from build123d import *

# Parameters (mm, degrees)
SKETCH1_W           = 330.2
SKETCH1_H           = 25.4
BOSS_EXTRUDE4_DEPTH = 50.8
SKETCH5_W           = 19.05
SKETCH5_H           = 44.45
CUT_EXTRUDE1_DEPTH  = 330.2
SKETCH7_W           = 25.4
SKETCH7_H           = 44.45
CUT_EXTRUDE4_DEPTH  = 31.496


with BuildPart() as part:
    # Sketch1 → Boss-Extrude4 (new body)
    with BuildSketch(Plane(origin=(0, 0, 0), x_dir=(1, 0, 0), z_dir=(0, 1, 0))):
        with Locations((-165.1, -12.7)):
            Rectangle(SKETCH1_W, SKETCH1_H)
    extrude(amount=BOSS_EXTRUDE4_DEPTH)

    # Sketch5 → Cut-Extrude1 (cut)
    with BuildSketch(Plane.ZY.offset(330.2)):
        with Locations((12.7, 25.4)):
            Rectangle(SKETCH5_W, SKETCH5_H)
    extrude(amount=-CUT_EXTRUDE1_DEPTH, mode=Mode.SUBTRACT)

    # Sketch7 → Cut-Extrude4 (cut)
    with BuildSketch(Plane(origin=(0, 0, 0), x_dir=(-1, 0, 0), z_dir=(0, 0, -1))):
        with Locations((317.5, 22.225)):
            Rectangle(SKETCH7_W, SKETCH7_H)
    extrude(amount=-CUT_EXTRUDE4_DEPTH, mode=Mode.SUBTRACT)


solid = part.part
Part model, mm, in its own coordinate system. A direction names the side the tool comes from. Round coordinates to 2 decimals unless told otherwise and drop trailing zeros. Order: outer loops, then holes, each group sorted by start corner. A loop starts at its lowest first (then second) coordinate and runs counter-clockwise, first axis right, second up. Notation, with made-up numbers: (10, 29) -> (20, 29) arc R19 ccw to (20, 39) -> close; hole circle Ø1 at (61, 3.5). An arc over 180 degrees is marked (long way). Put each result on its own line as item: value.
Q1. Pin check, flat tips, straight feed: pin 1 Ø12 at (y, z) = (25.5, 4.5) entering from -X; pin 2 Ø6 at (y, z) = (6.5, 19.5) entering from +X; pin 3 Ø2.5 at (x, z) = (-318, 23) entering from -Y. Stop position of each tip, or through.
From the geometry:
pin 1: stops at x = -304.8
pin 2: stops at x = 0
pin 3: stops at y = 44.45
Q2. Tool access for faces 1 (the face through (-167, 50.8, 13)), 2 (the face through (-304.8, 17, 23)), 3 (the face through (-167, 47.625, 13)): list every direction of +Z, -Z, +X, -X, +Y, -Y with a clear straight run to the whole face (end or side of a thin tool).
From the geometry:
face 1: +Z, -Z, +X, -X, +Y
face 2: +Z, -Z, -X, -Y
face 3: +X, -X
Q3. Band-saw the part on C-C (x = -291). Give the cut face in (y, z) (3 decimals), and give its area (3 significant figures).
From the geometry:
outline: (0, 0) -> (50.8, 0) -> (50.8, 25.4) -> (0, 25.4) -> close; hole (3.175, 3.175) -> (47.625, 3.175) -> (47.625, 22.225) -> (3.175, 22.225) -> close
area: 444 mm2
Q4. Wall check: line 1 (Z direction, x = -155, y = 23.5) (3 decimals); line 2 (Y direction, x = -259.5, z = 14) (3 decimals). Give the ranges that are in metal, low to high. Write a range as [from, to].
From the geometry:
line 1: z = [0, 3.175], [22.225, 25.4]
line 2: y = [0, 3.175], [47.625, 50.8]
Q5. Band-saw the part on B-B (y = 7). Give the cut face in (x, z) (3 decimals), and give its area (3 significant figures).
From the geometry:
outline: (-304.8, 0) -> (0, 0) -> (0, 3.175) -> (-304.8, 3.175) -> close; (-304.8, 22.225) -> (0, 22.225) -> (0, 25.4) -> (-304.8, 25.4) -> close
area: 1,940 mm2
Q6. Pull direction Z, two halves, no side cores. Call faces 4 (the face through (-167, 25, 0)), 5 (the face through (-167, 25, 22.225)), 6 (the face through (0, 27, 23)): pulls with the +Z half, pulls with the -Z half, needs draft (parallel to the pull), parting line crosses it, or undercut.
From the geometry:
face 4: pulls with the -Z half
face 5: undercut
face 6: needs draft
Q7. Band-saw the part on A-A (z = 18). Give the cut face in (x, y) (3 decimals).
From the geometry:
outline: (-330.2, 47.625) -> (0, 47.625) -> (0, 50.8) -> (-330.2, 50.8) -> close; (-304.8, 0) -> (0, 0) -> (0, 3.175) -> (-304.8, 3.175) -> close
